Autodesk Inventor part; units mm, degrees
ref_plane "YZ Plane" through (0, 0, 0) normal (1, 0, 0) x (0, 1, 0)
ref_plane "XZ Plane" through (0, 0, 0) normal (0, 1, 0) x (-1, 0, 0)
ref_plane "XY Plane" through (0, 0, 0) normal (0, 0, 1) x (1, 0, 0)
sketch "Эскиз1" plane through (0, 0, 0) normal (0, 0, 1) x (1, 0, 0)
  line L0 (-15, 0) -> (15, 0)
  line L1 (0, 120) -> (0, 125)
  line L2 (0, 125) -> (0, 180)
  line L3 (-48, 180) -> (48, 180)
  line L4 (-17, 125) -> (17, 125)
  line L5 (-15, 120) -> (15, 120)
  line L6 (0, 0) -> (0, 80)
  line L7 (0, 80) -> (0, 120)
  line L8 (-11.5, 80) -> (11.5, 80)
  line L9 (15, 0) -> (11.5, 80)
  line L10 (-15, 0) -> (-11.5, 80)
  arc A0 (17, 125) -> (11.5, 80) centre (149.09, 86.0196) ccw
  arc A1 (48, 180) -> (17, 125) centre (151.9429, 85.1776) ccw
  arc A2 (-11.5, 80) -> (-17, 125) centre (-149.09, 86.0196) ccw
  arc A3 (-17, 125) -> (-48, 180) centre (-151.9429, 85.1776) ccw
  dimension "d0" = 30
  dimension "d2" = 5
  dimension "d3" = 55
  dimension "d4" = 96
  dimension "d5" = 34
  dimension "d6" = 30
  dimension "d7" = 80
  dimension "d8" = 40
  dimension "d9" = 23
extrude "Выдавливание1" add sketch "Эскиз1" along normal blind 27
sketch "Эскиз2" plane through (0, 0, 0) normal (1, 0, 0) x (0, 1, 0)
  line L0 (80, 0) -> (0, 0)
  line L1 (0, 0) -> (0, 27)
  line L2 (80, 27) -> (0, 27)
  line L3 (80, 0) -> (80, 27)
  line L4 (125, 0) -> (80, 0)
  line L5 (80, 0) -> (80, 27)
  line L6 (125, 27) -> (80, 27)
  line L7 (125, 0) -> (125, 27)
  line L8 (180, 0) -> (125, 0)
  line L9 (125, 0) -> (125, 27)
  line L10 (180, 27) -> (125, 27)
  line L11 (180, 0) -> (180, 27)
  line L12 (125, 7) -> (125, 20)
  line L13 (125, 0) -> (125, 27)
  line L14 (125, 7) -> (0, 0)
  line L15 (0, 27) -> (125, 20)
  line L16 (125, 8) -> (125, 19)
  line L17 (180, 13.25) -> (180, 13.75)
  line L18 (180, 0) -> (180, 27)
  line L19 (125, 8) -> (180, 13.25)
  line L20 (180, 13.75) -> (125, 19)
  point P0 (125, 13.5)
  point P1 (125, 13.5)
  point P2 (180, 13.5)
  dimension "d12" = 13
  dimension "d13" = 11
  dimension "d14" = 0.5
extrude "Выдавливание2" cut sketch "Эскиз2" along normal mid plane 100 contours L1 L15 L3 L14 | L3 L15 L7 L14 | L7 L20 L11 L19 keep common part
chamfer "Фаска1" distance 1 angle 45 2 edges at (0, 125, 7) (0, 125, 20)
equation "\"d6\" = d0"
properties part number "bachi"
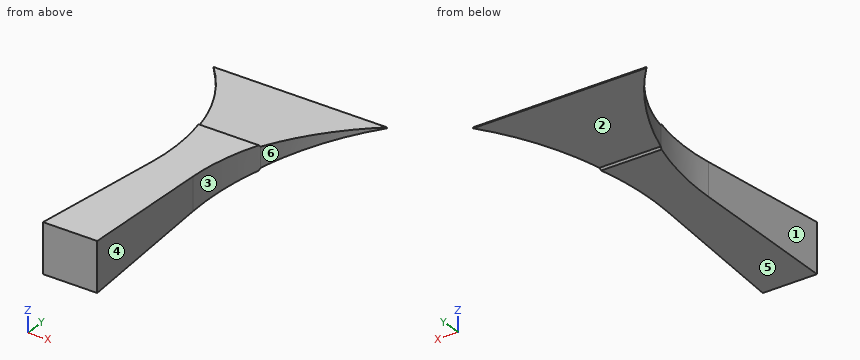
The listing builds one solid part. Answer for the finished solid, in the listing's coordinates (mm). Face numbers are marked on the shaded views. A direction names the side the tool comes from. Coordinates: 2 decimals unless noted, no trailing zeros. Loops run counter-clockwise (first coordinate to the right, second up) from the corner with the lowest first, then second, coordinate; pieces in that order, holes last. Notation, with made-up numbers: M 88,36 L 129,36 A25 ccw 129,58 Z; hole C 67.5,84 d10. An arc over 180 degrees is marked long. Answer as a JSON object with one key per item and string values. Group by question number.
Item 1: Section D-D (y = 93.5) is taken. Write down the section's boundary in (x, z).
Item 2: Section B-B (z = 9.75) is taken. Write down the section's boundary in (x, y).
Item 3: Which of the six approach directions +Z, -Z, +X, -X, +Y, -Y give full straight-line access (tool end or side, diameter ignored) to the marked faces 1, 2 and 3?
Item 4: Consider L1, parallel to Z at x = -6.5, y = 131; L2, parallel to X at y = 94, z = 12.5; L3, parallel to Z at x = -16, y = 137.5. Determine where each line is inside the solid, lowest interval first.
Item 5: Section C-C (y = 159) is taken. Write down the section's boundary in (x, z), and give its area (3 significant figures).
Item 6: Determine the mould class of the marked faces 4, 5 and 6 for opening direction Y: +Y half, -Y half, draft (parallel to the pull), parting line (faces both ways), or undercut.
Item 7: Each of these flat-tipped pins is pushed along its axis until it touches: P1, Ø1.5, axis at x = 11, y = 116.5, coming from the -Z side; P2, Ø1, axis at x = -34.5, z = 11.5, coming from the -Y side; P3, Ø4, axis at y = 152, z = 15, coming from the -X side. Where does it stop, or does it pass through?
Solved:
{
 "1": {"outline": "M -11.57,5.24 L 11.57,5.24 L 11.57,21.76 L -11.57,21.76 Z"},
 "2": {"outline": "M -23.83,143.33 A140.7 cw -17,125 A137.72 cw -11.5,80 L -15,0 L 15,0 L 11.5,80 A137.72 cw 17,125 A140.7 cw 23.83,143.33 Z"},
 "3": {"face 1": "+Z, -Z, -X", "face 2": "-Z, +X, -X, +Y", "face 3": "+Z, -Z, +X"},
 "4": {"L1": "z = 8.57 to 18.43", "L2": "x = -11.6 to 11.6", "L3": "z = 9.19 to 17.81"},
 "5": {"outline": "M -32.17,11.25 L 32.17,11.25 L 32.17,15.75 L -32.17,15.75 Z", "area": "290 mm2"},
 "6": {"face 4": "undercut", "face 5": "+Y half", "face 6": "-Y half"},
 "7": {"P1": "stops at z = 6.48", "P2": "stops at y = 161.89", "P3": "stops at x = -29.23"}
}
